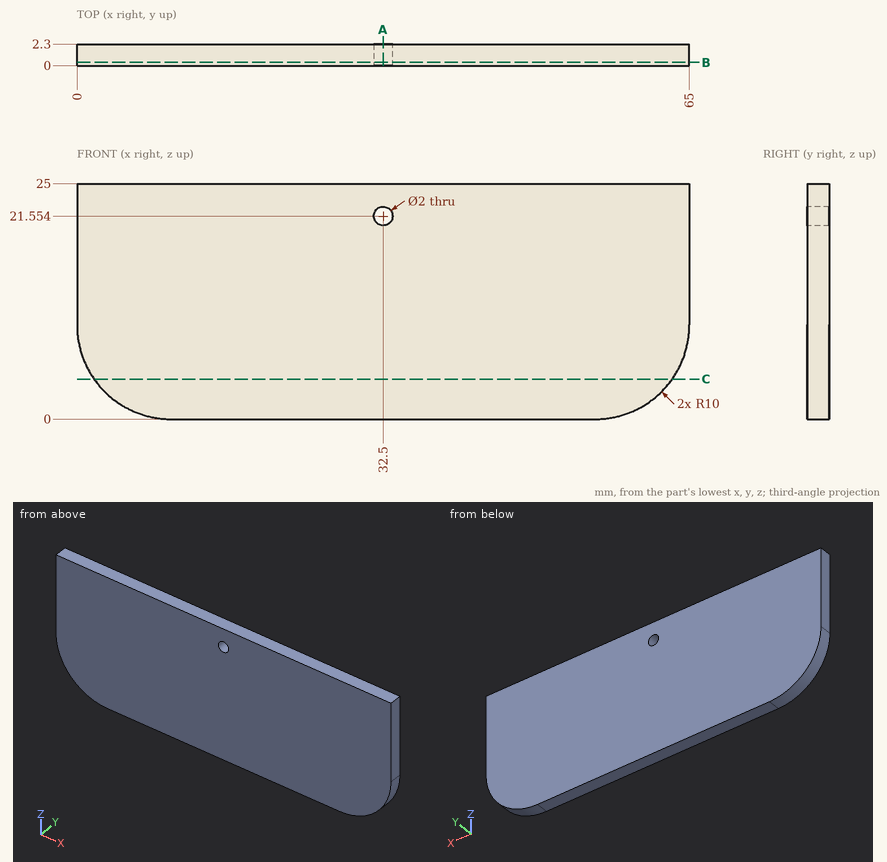
Design review of the part shown in the three views and the two pictorial views. Dimensions are in mm from the part's minimum x, y and z. Coordinates: 2 decimals unless noted, no trailing zeros. Loops run counter-clockwise (first coordinate to the right, second up) from the corner with the lowest first, then second, coordinate; pieces in that order, holes last. Notation, with made-up numbers: M 87,-20 L 123,-20 A15 cw 123,-2 Z; hole C 76,33.5 d3. An arc over 180 degrees is marked long. Put each result on its own line as item: value. Start each with the question number.
Q1. Add section C-C (z = 4.25). Write out the cut boundary in (x, y).
Q2. Wall thickness on line 1 (Z direction, x = 32.5, y = 1.05) (1 decimal); line 2 (X direction, y = 1.65, z = 21); line 3 (X direction, y = 0.5, z = 3.75) (1 decimal): over which ranges is each line inside the solid? List them lowest first.
Q3. Add section A-A (x = 32.5). Write out the cut boundary in (y, z) (1 decimal).
Q4. Add section B-B (y = 0.35). Write out the cut boundary in (x, z) (1 decimal), and give its area (3 significant figures).
Answers:
1. outline: M 1.82,0 L 63.18,0 L 63.18,2.3 L 1.82,2.3 Z
2. line 1: z = 0 to 20.6, 22.6 to 25
2. line 2: x = 0 to 31.67, 33.33 to 65
2. line 3: x = 2.2 to 62.8
3. outline: M 0,0 L 2.3,0 L 2.3,20.6 L 0,20.6 Z; M 0,22.6 L 2.3,22.6 L 2.3,25 L 0,25 Z
4. outline: M 0,10 A10 ccw 10,0 L 55,0 A10 ccw 65,10 L 65,25 L 0,25 Z; hole C 32.5,21.6 d2
4. area: 1,580 mm^2
